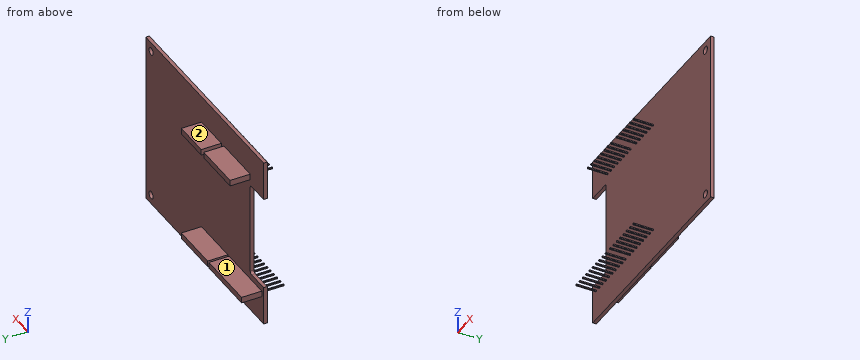
from build123d import *

# Parameters (mm, degrees)
SZKIC1_R                    = 1.6
DODANIE_WYCI_GNI_CIE1_DEPTH = 1.5
SZKIC2_W                    = 15.5
SZKIC2_H                    = 2.5
SZKIC2_W_2                  = 20.5
SZKIC2_W_3                  = 25.5
DODANIE_WYCI_GNI_CIE2_DEPTH = 8.5
SZKIC3_W                    = 0.5
SZKIC3_H                    = 0.5
DODANIE_WYCI_GNI_CIE3_DEPTH = 8.5


with BuildPart() as part:
    # Szkic1 → Dodanie-wyciągnięcie1 (new body)
    with BuildSketch(Plane(origin=(0, 0, 0), x_dir=(1, 0, 0), z_dir=(0, 1, 0))):
        with BuildLine():
            Line((-46, 36.5), (46, 36.5))
            Line((46, 36.5), (46, -36.5))
            Line((46, -36.5), (-46, -36.5))
            Line((-46, -36.5), (-46, -20))
            Line((-46, -20), (-36.5, -20))
            ThreePointArc((-36.5, -20), (-35.792893219, -19.707106781), (-35.5, -19))
            Line((-35.5, -19), (-35.5, 19))
            ThreePointArc((-35.5, 19), (-35.792893219, 19.707106781), (-36.5, 20))
            Line((-36.5, 20), (-46, 20))
            Line((-46, 20), (-46, 36.5))
        make_face()
        with Locations((41.86, 32.6)):
            Circle(SZKIC1_R, mode=Mode.SUBTRACT)
        with Locations((41.86, -32.6)):
            Circle(SZKIC1_R, mode=Mode.SUBTRACT)
    extrude(amount=DODANIE_WYCI_GNI_CIE1_DEPTH)

    # Szkic2 → Dodanie-wyciągnięcie2 (add)
    with BuildSketch(Plane(origin=(0, 1.5, 0), x_dir=(1, 0, 0), z_dir=(0, 1, 0))):
        with Locations((-5.25, -23.75)):
            Rectangle(SZKIC2_W, SZKIC2_H)
        with Locations((-25.25, -23.75)):
            Rectangle(SZKIC2_W_2, SZKIC2_H)
        with Locations((-7.75, 23.75)):
            Rectangle(SZKIC2_W_2, SZKIC2_H)
        with Locations((-31.75, 23.75)):
            Rectangle(SZKIC2_W_3, SZKIC2_H)
    extrude(amount=DODANIE_WYCI_GNI_CIE2_DEPTH)

    # Szkic3 → Dodanie-wyciągnięcie3 (add)
    with BuildSketch(Plane.XZ):
        with Locations((-43.25, -23.75)):
            Rectangle(SZKIC3_W, SZKIC3_H)
        with Locations((-40.694444444, -23.75)):
            Rectangle(SZKIC3_W, SZKIC3_H)
        with Locations((-38.138888889, -23.75)):
            Rectangle(SZKIC3_W, SZKIC3_H)
        with Locations((-35.583333333, -23.75)):
            Rectangle(SZKIC3_W, SZKIC3_H)
        with Locations((-33.027777778, -23.75)):
            Rectangle(SZKIC3_W, SZKIC3_H)
        with Locations((-30.472222222, -23.75)):
            Rectangle(SZKIC3_W, SZKIC3_H)
        with Locations((-27.916666667, -23.75)):
            Rectangle(SZKIC3_W, SZKIC3_H)
        with Locations((-25.361111111, -23.75)):
            Rectangle(SZKIC3_W, SZKIC3_H)
        with Locations((-22.805555556, -23.75)):
            Rectangle(SZKIC3_W, SZKIC3_H)
        with Locations((-20.25, -23.75)):
            Rectangle(SZKIC3_W, SZKIC3_H)
        with Locations((-16.75, -23.75)):
            Rectangle(SZKIC3_W, SZKIC3_H)
        with Locations((-14.178571429, -23.75)):
            Rectangle(SZKIC3_W, SZKIC3_H)
        with Locations((-11.607142857, -23.75)):
            Rectangle(SZKIC3_W, SZKIC3_H)
        with Locations((-9.035714286, -23.75)):
            Rectangle(SZKIC3_W, SZKIC3_H)
        with Locations((-6.464285714, -23.75)):
            Rectangle(SZKIC3_W, SZKIC3_H)
        with Locations((-3.892857143, -23.75)):
            Rectangle(SZKIC3_W, SZKIC3_H)
        with Locations((-1.321428571, -23.75)):
            Rectangle(SZKIC3_W, SZKIC3_H)
        with Locations((1.25, -23.75)):
            Rectangle(SZKIC3_W, SZKIC3_H)
        with Locations((-34.25, 23.75)):
            Rectangle(SZKIC3_W, SZKIC3_H)
        with Locations((-31.678571432, 23.750167466)):
            Rectangle(SZKIC3_W, SZKIC3_H)
        with Locations((-29.107142864, 23.750334931)):
            Rectangle(SZKIC3_W, SZKIC3_H)
        with Locations((-26.535714297, 23.750502397)):
            Rectangle(SZKIC3_W, SZKIC3_H)
        with Locations((-23.964285729, 23.750669862)):
            Rectangle(SZKIC3_W, SZKIC3_H)
        with Locations((-21.392857161, 23.750837328)):
            Rectangle(SZKIC3_W, SZKIC3_H)
        with Locations((-18.821428593, 23.751004794)):
            Rectangle(SZKIC3_W, SZKIC3_H)
        Polygon((-16, 23.501172259), (-16, 24), (-16.000000025, 24.001172259), (-16.500000025, 24.001172259), (-16.500000025, 23.501172259), align=None)
        with Locations((-11.75, 23.75)):
            Rectangle(SZKIC3_W, SZKIC3_H)
        with Locations((-9.15, 23.75)):
            Rectangle(SZKIC3_W, SZKIC3_H)
        with Locations((-6.55, 23.75)):
            Rectangle(SZKIC3_W, SZKIC3_H)
        with Locations((-3.95, 23.75)):
            Rectangle(SZKIC3_W, SZKIC3_H)
        with Locations((-1.35, 23.75)):
            Rectangle(SZKIC3_W, SZKIC3_H)
        with Locations((1.25, 23.75)):
            Rectangle(SZKIC3_W, SZKIC3_H)
    extrude(amount=DODANIE_WYCI_GNI_CIE3_DEPTH)


solid = part.part
Input: part model. Units: mm. Frame: model coordinates. Face numbers are marked on the shaded views. A direction names the side the tool comes from. Give positions to 0.01 mm unless a question says otherwise; leave off trailing zeros. Order: outer loops, then holes, each group sorted by start corner. A loop starts at its lowest first (then second) coordinate and runs counter-clockwise, first axis right, second up.
Q1. Contact query for flat-ended pins moving along their axis: pin 1 Ø12 at (x, z) = (25, 5.5) entering from -Y; pin 2 Ø0.6 at (x, y) = (-4, -6) entering from -Z; pin 3 Ø0.6 at (x, y) = (-6.5, -5) entering from +Z. Output: stop coordinate, or through.
Checked values:
pin 1: stops at y = 0
pin 2: stops at z = -24
pin 3: stops at z = 24
Q2. Set-up query: the marked faces 1 and 2. Return all of +Z, -Z, +X, -X, +Y, -Y with unobstructed straight access to the full face (end or side cutting, diameter ignored); none if empty.
Checked values:
face 1: +X, -X, +Y
face 2: +Z, +X, -X, +Y
Q3. Section C-C on z = 32.6. Output: boundary loops of the cut face in (x, y).
Checked values:
outline: (-46, 0) - (40.26, 0) - (40.26, 1.5) - (-46, 1.5) - close; (43.46, 0) - (46, 0) - (46, 1.5) - (43.46, 1.5) - close
Q4. Ray query, probe 1 along Z at (x, y) = (41.86, 1.2); probe 2 along X at (y, z) = (0.9, 32.6); probe 3 along Y at (x, z) = (10.5, -27.5). Return the intervals inside material, ascending.
Checked values:
probe 1: z = -36.5 to -34.2, -31 to 31, 34.2 to 36.5
probe 2: x = -46 to 40.26, 43.46 to 46
probe 3: y = 0 to 1.5
Q5. Section B-B on y = 8.25. Output: boundary loops of the cut face in (x, z), and give its area (3 significant figures).
Checked values:
outline: (-44.5, -25) - (-19, -25) - (-19, -22.5) - (-44.5, -22.5) - close; (-35.5, 22.5) - (-15, 22.5) - (-15, 25) - (-35.5, 25) - close; (-18, -25) - (2.5, -25) - (2.5, -22.5) - (-18, -22.5) - close; (-13, 22.5) - (2.5, 22.5) - (2.5, 25) - (-13, 25) - close
area: 205 mm2
Q6. Section A-A on x = 41.86. Output: boundary loops of the cut face in (y, z).
Checked values:
outline: (0, -36.5) - (1.5, -36.5) - (1.5, -34.2) - (0, -34.2) - close; (0, -31) - (1.5, -31) - (1.5, 31) - (0, 31) - close; (0, 34.2) - (1.5, 34.2) - (1.5, 36.5) - (0, 36.5) - close
Q7. Section D-D on y = -1.75. State how many separate pieces and enclosed holes the cut face has, and give its area (3 significant figures).
Checked values:
separate pieces: 32
enclosed holes: 0
area: 8.00 mm2
